Check sheet for the modelled part. Datum: model origin and axes. Units: mm. A direction names the side the tool comes from. Coordinates: 2 decimals unless noted, no trailing zeros. Loops run counter-clockwise (first coordinate to the right, second up) from the corner with the lowest first, then second, coordinate; pieces in that order, holes last.
from build123d import *

# Parameters (mm, degrees)
F4_DEPTH  = 4.000005
F1_R      = 2.399995
F5_DEPTH  = 1.599999
F2_R      = 2.368695
F6_DEPTH  = 25.4
F6_FACE_R = 2.368695
F7_DEPTH  = 1.599999
F3_W      = 0.8
F3_H      = 0.8
F8_DEPTH  = 1.599999


with BuildPart() as f4:
    # F0 (on Front) → F4 (new body, symmetric)
    with BuildSketch(Plane.XZ):
        Polygon((3.200006, 0), (0, 0), (-3.200006, 0), (-3.200006, -9.5758), (3.200006, -9.5758), align=None)
    extrude(amount=F4_DEPTH, both=True)

    # F1 (on Top) → F5 (join)
    with BuildSketch(Plane.XY):
        Circle(F1_R)
    extrude(amount=F5_DEPTH)

    # F2 (on Top) → F6 (cut)
    with BuildSketch(Plane.XY):
        Circle(F2_R)
    extrude(amount=-F6_DEPTH, mode=Mode.SUBTRACT)

    # F6_face (on face) → F7 (join)
    with BuildSketch(Plane(origin=(0, 0, 0), x_dir=(1, 0, 0), z_dir=(0, 0, -1))):
        Circle(F6_FACE_R)
    extrude(amount=F7_DEPTH)

    # F3 (on Top) → F8 (cut)
    with BuildSketch(Plane.XY):
        Rectangle(F3_W, F3_H)
    extrude(amount=-F8_DEPTH, mode=Mode.SUBTRACT)


solid = f4.part
(1) Section check D-D, the plane x = 1.5. Enter the section's corners in (y, z), plus the area to 3 significant figures.
(2) Gauge pin test, flat end, axial feed: P1, Ø1.4, axis at x = -1, y = -0.5, coming from the -Z side. Record the tip position at first contact, or that the pin passes through.
(3) Scan lines: line 1 along X through (y, z) = (0, -4.25); line 2 along Y through (x, z) = (0, -6.5); line 3 along Z through (x, y) = (-2, -3). Record each from-to range of solid material in increasing order.
(4) Set-up check for faces 1 (the face through (0, -3, -9.576)), 2 (the face through (0, -3, 0)): record each of +Z, -Z, +X, -X, +Y, -Y from which the full face is reachable in a straight line by a thin tool's end or side.
(5) Section check C-C, the plane x = 0. Enter the section's corners in (y, z), plus the area to 3 significant figures.
(6) Section check A-A, the plane z = -3.5. Enter the section's corners in (x, y), plus the area to 3 significant figures.
(7) Draft check along Y on faces 3 (the face through (-1.905, -1.46, 0.789)), 4 (the face through (-1, 0, -1.6)), 5 (the face through (-1.746, 1.601, -5.532)), 6 (the face through (3.2, 0, -5)). Enter one of: pulls with the +Y half, pulls with the -Y half, needs draft (parallel to the pull), parting line crosses it, or undercut.
(8) Section check B-B, the plane y = 0. Enter the section's corners in (x, z), plus the area to 3 significant figures.
Determined:
1. outline: (-4, -9.58) - (-1.83, -9.58) - (-1.83, -1.6) - (1.83, -1.6) - (1.83, -9.58) - (4, -9.58) - (4, 0) - (1.87, 0) - (1.87, 1.6) - (-1.87, 1.6) - (-1.87, 0) - (-4, 0) - close
1. area: 53.4 mm2
2. P1: stops at z = -1.6
3. line 1: x = -3.2 to -2.37, 2.37 to 3.2
3. line 2: y = -4 to -2.37, 2.37 to 4
3. line 3: z = -9.58 to 0
4. face 1: -Z, +X, -X, +Y, -Y
4. face 2: +Z
5. outline: (-4, -9.58) - (-2.37, -9.58) - (-2.37, -1.6) - (-0.4, -1.6) - (-0.4, 0) - (0.4, 0) - (0.4, -1.6) - (2.37, -1.6) - (2.37, -9.58) - (4, -9.58) - (4, 0) - (2.4, 0) - (2.4, 1.6) - (-2.4, 1.6) - (-2.4, 0) - (-4, 0) - close
5. area: 45.2 mm2
6. outline: (-3.2, -4) - (3.2, -4) - (3.2, 4) - (-3.2, 4) - close; hole circle Ø4.74 at (0, 0)
6. area: 33.6 mm2
7. face 3: parting line crosses it
7. face 4: undercut
7. face 5: undercut
7. face 6: needs draft
8. outline: (-3.2, -9.58) - (-2.37, -9.58) - (-2.37, -1.6) - (-0.4, -1.6) - (-0.4, 0) - (0.4, 0) - (0.4, -1.6) - (2.37, -1.6) - (2.37, -9.58) - (3.2, -9.58) - (3.2, 0) - (2.4, 0) - (2.4, 1.6) - (-2.4, 1.6) - (-2.4, 0) - (-3.2, 0) - close
8. area: 29.9 mm2
